Can you work these out from the drawing? Everything is in mm from the part's minimum corner. A direction names the side the tool comes from. Round coordinates to 2 decimals unless told otherwise and drop trailing zeros. Write each loop counter-clockwise with the first axis right and the second up, starting at its lowest first coordinate (ties: lowest second). Pieces come first, ordered by that corner, then holes. Notation, with made-up numbers: (60.25, -5) -> (90.25, -5) arc R32 ccw to (90.25, 29) -> close; hole circle Ø8 at (82, 74). An arc over 180 degrees is marked (long way). Answer as CSV lines item,"result".
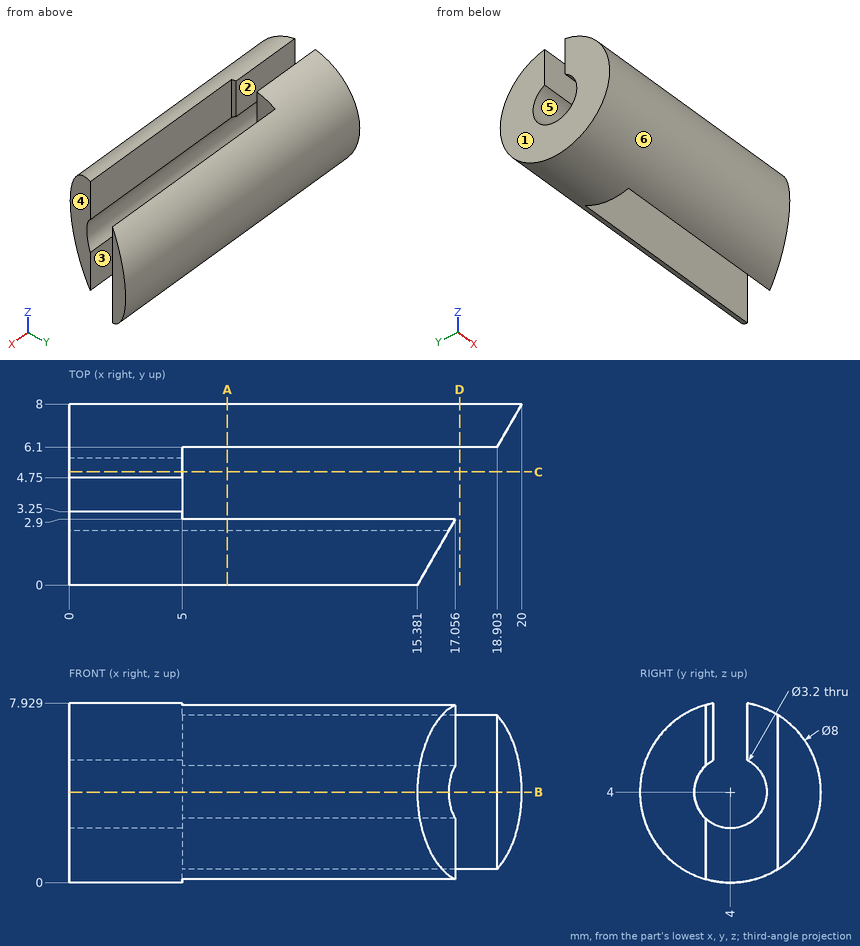
Item 1: Suppose I cut it at A-A, the plane x = 7. List the corners of the cut face in (y, z) for me (1 decimal).
Results found:
outline,"(2.9, 0.2) -> (2.9, 2.8) arc R1.6 cw to (2.9, 5.2) -> (2.9, 7.8) arc R4 ccw to start; (6.1, 0.6) arc R4 ccw to (6.1, 7.4) -> close"
Item 2: Suppose I cut it at D-D, the plane x = 17.25. List the corners of the cut face in (y, z) for me (1 decimal).
Results found:
outline,"(6.1, 0.6) arc R4 ccw to (6.1, 7.4) -> close"
Item 3: Suppose I cut it at B-B, the plane z = 4. List the corners of the cut face in (x, y) for me.
Results found:
outline,"(0, 0) -> (15.38, 0) -> (16.77, 2.4) -> (0, 2.4) -> close; (0, 5.6) -> (5, 5.6) -> (5, 6.1) -> (18.9, 6.1) -> (20, 8) -> (0, 8) -> close"
Item 4: Will these pins go through, and if not, where does the flat tip stop? pin 1 (3 mm diameter, centred on x = 3.5, z = 6.5, fed in from +Y); pin 2 (1 mm diameter, centred on x = 8, y = 6.5, fed in from +Z); pin 3 (1.5 mm diameter, centred on x = 5, z = 6, fed in from -Y).
Results found:
pin 1,"stops at y = 7.87"
pin 2,"stops at z = 7.4"
pin 3,"stops at y = 0.2"
Item 5: If we mould it in two halves opening along Z, with no side actions, what happens to the marked faces 4, 5 and 6? For each: pulls with the +Z half, pulls with the -Z half, needs draft (parallel to the pull), parting line crosses it, or undercut.
Results found:
face 4,"needs draft"
face 5,"undercut"
face 6,"parting line crosses it"
Item 6: I need wall thicknesses on L1, parallel to Y at x = 11.75, z = 4; L2, parallel to Y at x = 4, z = 4; L3, parallel to X at y = 3, z = 1.75. Which ranges of each line are inside material? Lowest first, please.
Results found:
L1,"y = 0 to 2.4, 6.1 to 8"
L2,"y = 0 to 2.4, 5.6 to 8"
L3,"x = 0 to 5"
Item 7: For the marked faces 1, 2 and 3, which set-ups out of +Z, -Z, +X, -X, +Y, -Y let a thin tool reach every point of the face, with its end or its side?
Results found:
face 1,"+Z, -Z, -X, +Y, -Y"
face 2,"+Z, +X, -X"
face 3,"+Z, -Z, +X"
Item 8: Suppose I cut it at C-C, the plane y = 5. List the corners of the cut face in (x, z) for me.
Results found:
outline,"(0, 0.13) -> (5, 0.13) -> (5, 2.75) -> (0, 2.75) -> close; (0, 5.25) -> (5, 5.25) -> (5, 7.87) -> (0, 7.87) -> close"
